Read the model definition and answer for the solid it produces. Units are mm, in the model's axes. Face numbers are marked on the shaded views. Give positions to 0.01 mm unless a question says otherwise; leave off trailing zeros. Order: outer loops, then holes, each group sorted by start corner. A loop starts at its lowest first (then second) coordinate and runs counter-clockwise, first axis right, second up.
Item 1: A cutting plane is placed at B-B (x = 32.5). Write down the section's boundary in (y, z).
Item 2: Given pin 1 Ø4 at (y, z) = (-10.5, 19.7) entering from -X; pin 2 Ø5 at (y, z) = (21.5, -8) entering from +X; pin 3 Ø12 at (x, z) = (32.5, 0) entering from -Y, each flat-ended and moving along its own axis, determine where each tip first touches the part or whether it passes through.
Item 3: Find the intervals of material crossed by line 1 along Y through (x, z) = (2.95, 19.7) (3 decimals); line 2 along Z through (x, y) = (1, 19); line 3 along Y through (x, z) = (-24.5, -26.1), in increasing order.
Item 4: The mould has two halves that part along Y. Classify the marked faces 1, 2, 3 and 4: +Y half, -Y half, draft (parallel to the pull), parting line (faces both ways), or undercut.
Item 5: A cutting plane is placed at D-D (y = -20). Write down the section's boundary in (x, z), plus the area to 3 significant figures.
Item 6: A cutting plane is placed at C-C (z = 3.5). Write down the section's boundary in (x, y).
Item 7: A cutting plane is placed at A-A (y = 19.7). Write down the section's boundary in (x, z) (3 decimals), plus the area to 3 significant figures.
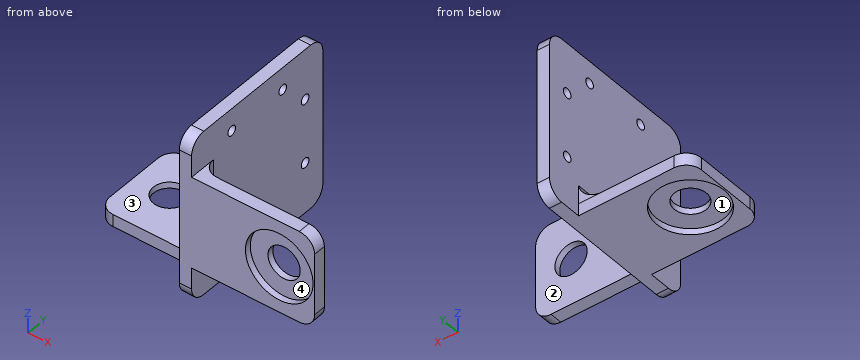
from build123d import *

# Parameters (mm, degrees)
SKETCH1_W            = 54
SKETCH1_H            = 54
BOSS_EXTRUDE1_DEPTH  = 4
FILLET1_R            = 5
SKETCH2_W            = 30
SKETCH2_H            = 4
BOSS_EXTRUDE2_DEPTH  = 3
SKETCH3_W            = 30
SKETCH3_H            = 4
BOSS_EXTRUDE3_DEPTH  = 37
SKETCH4_W            = 4
SKETCH4_H            = 30.000186299
BOSS_EXTRUDE6_DEPTH  = 3
SKETCH6_W            = 4
SKETCH6_H            = 30.000186299
BOSS_EXTRUDE7_DEPTH  = 33
FILLET2_R            = 5
SKETCH7_R            = 1.25
CUT_EXTRUDE1_DEPTH   = 75.706090782
SKETCH8_R            = 1.25
CUT_EXTRUDE2_DEPTH   = 75.706090782
SKETCH9_R            = 1.575
CUT_EXTRUDE3_DEPTH   = 56.299186251
SKETCH10_R           = 1.575
CUT_EXTRUDE4_DEPTH   = 56.299186251
FILLET6_R            = 5
SKETCH11_R           = 1.575
CUT_EXTRUDE5_DEPTH   = 59.258046655
SKETCH12_R           = 1.575
CUT_EXTRUDE6_DEPTH   = 33
BOSS_EXTRUDE10_DEPTH = 30
SKETCH15_R           = 11
CUT_EXTRUDE7_DEPTH   = 2
SKETCH16_R           = 5.25
CUT_EXTRUDE8_DEPTH   = 2
SKETCH17_R           = 11
CUT_EXTRUDE9_DEPTH   = 2
SKETCH18_R           = 5.25
CUT_EXTRUDE10_DEPTH  = 2


with BuildPart() as part:
    # Sketch1 → Boss-Extrude1 (new body)
    with BuildSketch(Plane(origin=(0, 0, 0), x_dir=(0, 0, -1), z_dir=(1, 0, 0))):
        Rectangle(SKETCH1_W, SKETCH1_H)
    extrude(amount=BOSS_EXTRUDE1_DEPTH)

    # Fillet1
    fillet1_edges = [part.edges().sort_by_distance(p)[0] for p in [
        (2, -27, -27),
        (2, -27, 27),
        (2, 27, 27),
        (2, 27, -27),
    ]]
    fillet(fillet1_edges, radius=FILLET1_R)

    # Sketch2 → Boss-Extrude2 (add)
    with BuildSketch(Plane(origin=(4, 0, 0), x_dir=(0, 0, -1), z_dir=(1, 0, 0))):
        with Locations((0.003473607, -25)):
            Rectangle(SKETCH2_W, SKETCH2_H)
    extrude(amount=BOSS_EXTRUDE2_DEPTH)

    # Sketch3 → Boss-Extrude3 (add)
    with BuildSketch(Plane(origin=(7, 0, 0), x_dir=(0, 0, -1), z_dir=(1, 0, 0))):
        with Locations((0.003473607, -25)):
            Rectangle(SKETCH3_W, SKETCH3_H)
    extrude(amount=BOSS_EXTRUDE3_DEPTH)

    # Sketch4 → Boss-Extrude6 (add)
    with BuildSketch(Plane.ZY):
        with Locations((-25, 0.003724222)):
            Rectangle(SKETCH4_W, SKETCH4_H)
    extrude(amount=BOSS_EXTRUDE6_DEPTH)

    # Sketch6 → Boss-Extrude7 (add)
    with BuildSketch(Plane.ZY.offset(3)):
        with Locations((-25, 0.003724222)):
            Rectangle(SKETCH6_W, SKETCH6_H)
    extrude(amount=BOSS_EXTRUDE7_DEPTH)

    # Fillet2
    fillet2_edges = [part.edges().sort_by_distance(p)[0] for p in [
        (44, -25, 14.996526393),
        (44, -25, -15.003473607),
        (-36, -14.996368927, -25),
        (-36, 15.003817372, -25),
    ]]
    fillet(fillet2_edges, radius=FILLET2_R)

    # Sketch7 → Cut-Extrude1 (cut, through all)
    with BuildSketch(Plane(origin=(0, 0, -27), x_dir=(-1, 0, 0), z_dir=(0, 0, -1))):
        with Locations((24.5, 0)):
            Circle(SKETCH7_R)
    extrude(amount=-CUT_EXTRUDE1_DEPTH, mode=Mode.SUBTRACT)

    # Sketch8 → Cut-Extrude2 (cut, through all)
    with BuildSketch(Plane(origin=(0, -27, 0), x_dir=(-1, 0, 0), z_dir=(0, -1, 0))):
        with Locations(Location((-32.5, 0, 0), (0, 0, 90))):
            Circle(SKETCH8_R)
    extrude(amount=-CUT_EXTRUDE2_DEPTH, mode=Mode.SUBTRACT)

    # Sketch9 → Cut-Extrude3 (cut, through all)
    with BuildSketch(Plane(origin=(4, 0, 0), x_dir=(0, 0, -1), z_dir=(1, 0, 0))):
        with Locations((-10.5, 19.7)):
            Circle(SKETCH9_R)
    extrude(amount=-CUT_EXTRUDE3_DEPTH, mode=Mode.SUBTRACT)

    # Sketch10 → Cut-Extrude4 (cut, through all)
    with BuildSketch(Plane(origin=(4, 0, 0), x_dir=(0, 0, -1), z_dir=(1, 0, 0))):
        with Locations((10.5, 19.7)):
            Circle(SKETCH10_R)
    extrude(amount=-CUT_EXTRUDE4_DEPTH, mode=Mode.SUBTRACT)

    # Fillet6
    fillet6_edges = [part.edges().sort_by_distance(p)[0] for p in [
        (4, -23, -0.003473607),
    ]]
    fillet(fillet6_edges, radius=FILLET6_R)

    # Sketch11 → Cut-Extrude5 (cut, through all)
    with BuildSketch(Plane.ZY):
        with Locations((19.7, 10.5)):
            Circle(SKETCH11_R)
    extrude(amount=-CUT_EXTRUDE5_DEPTH, mode=Mode.SUBTRACT)

    # Sketch12 → Cut-Extrude6 (cut)
    with BuildSketch(Plane.ZY):
        with Locations((19.7, -10.5)):
            Circle(SKETCH12_R)
    extrude(amount=-CUT_EXTRUDE6_DEPTH, mode=Mode.SUBTRACT)

    # Sketch14 → Boss-Extrude10 (add)
    with BuildSketch(Plane(origin=(0, -14.996368927, 0), x_dir=(-1, 0, 0), z_dir=(0, -1, 0))):
        with BuildLine():
            Line((6.771773058, 23), (0, 23))
            Line((0, 23), (0, 17.043091053))
            add(Edge.make_bspline(
                [(0, 17.043091053), (0.522042102, 20.003738935), (3.432344379, 22.411168624), (6.771773058, 23)],
                knots=[0, 0, 0, 0, 1, 1, 1, 1], degree=3))
        make_face()
    extrude(amount=-BOSS_EXTRUDE10_DEPTH)

    # Sketch15 → Cut-Extrude7 (cut)
    with BuildSketch(Plane(origin=(0, -27, 0), x_dir=(-1, 0, 0), z_dir=(0, -1, 0))):
        with Locations(Location((-32.5, 0, 0), (0, 0, 90))):
            Circle(SKETCH15_R)
    extrude(amount=-CUT_EXTRUDE7_DEPTH, mode=Mode.SUBTRACT)

    # Sketch16 → Cut-Extrude8 (cut)
    with BuildSketch(Plane(origin=(0, -23, 0), x_dir=(1, 0, 0), z_dir=(0, 1, 0))):
        with Locations(Location((32.5, 0, 0), (0, 0, 270))):
            Circle(SKETCH16_R)
    extrude(amount=-CUT_EXTRUDE8_DEPTH, mode=Mode.SUBTRACT)

    # Sketch17 → Cut-Extrude9 (cut)
    with BuildSketch(Plane(origin=(0, 0, -27), x_dir=(-1, 0, 0), z_dir=(0, 0, -1))):
        with Locations((24.5, 0)):
            Circle(SKETCH17_R)
    extrude(amount=-CUT_EXTRUDE9_DEPTH, mode=Mode.SUBTRACT)

    # Sketch18 → Cut-Extrude10 (cut)
    with BuildSketch(Plane.XY.offset(-23)):
        with Locations((-24.5, 0)):
            Circle(SKETCH18_R)
    extrude(amount=-CUT_EXTRUDE10_DEPTH, mode=Mode.SUBTRACT)


solid = part.part
Response values:
1. outline: (-27, -15) - (-23, -15) - (-23, -5.25) - (-25, -5.25) - (-25, -11) - (-27, -11) - close; (-27, 11) - (-25, 11) - (-25, 5.25) - (-23, 5.25) - (-23, 15) - (-27, 15) - close
2. pin 1: stops at x = 0
2. pin 2: stops at x = 4
2. pin 3: stops at y = -25
3. line 1: y = -27 to -12.075, -8.925 to 8.925, 12.075 to 27
3. line 2: z = -27 to -11.91, -9.09 to 9.09, 11.91 to 27
3. line 3: y = -15 to -11, 11 to 15
4. face 1: undercut
4. face 2: +Y half
4. face 3: draft
4. face 4: -Y half
5. outline: (0, -27) - (4, -27) - (4, -15) - (4.42, -15) - (4.42, 15) - (4, 15) - (4, 27) - (0, 27) - close
5. area: 229 mm2
6. outline: (0, -27) - (22.07, -27) - (22.07, -25) - (28.59, -25) - (28.59, -23) - (9, -23) arc R5 cw to (4, -18) - (4, 27) - (0, 27) - close; (36.41, -25) - (42.93, -25) - (42.93, -27) - (44, -27) - (44, -23) - (36.41, -23) - close
7. outline: (0, -27) - (4, -27) - (4, -12.075) - (0, -12.075) - close; (0, -8.925) - (4, -8.925) - (4, 8.925) - (0, 8.925) - close; (0, 12.075) - (4, 12.075) - (4, 27) - (0, 27) - close
7. area: 191 mm2
